Build history of the part. All positions in model axes, mm. A direction names the side the tool comes from. Round coordinates to 2 decimals unless told otherwise and drop trailing zeros. Order: outer loops, then holes, each group sorted by start corner. A loop starts at its lowest first (then second) coordinate and runs counter-clockwise, first axis right, second up. Notation, with made-up numbers: (-16, 48.25) -> (-1, 48.25) arc R22 cw to (-1, 84.25) -> close; hole circle Ø6 at (-5.5, -24.75). An arc over 180 degrees is marked (long way). Use a Markdown table: item, result. Add a question column.
Item 1: Slice it at B-B, the plane x = 64.4. Give the cut face in (y, z).
Item 2: Probe L1, parallel to X at y = 5.25, z = 0; L2, parallel to Z at x = 0, y = 7.15; L3, parallel to Z at x = -29, y = 5. List the from-to ranges inside material, lowest first.
Item 3: Slice it at C-C, the plane y = 2.5. State how many separate pieces and enclosed holes the cut face has, plus the area to 3 significant figures.
Item 4: Pin check, flat tips, straight feed: pin 1 (7 mm diameter, centred on x = 0, z = -64.4, fed in from -Y); pin 2 (1.5 mm diameter, centred on x = -7.5, y = 3.5, fed in from -Z); pin 3 (23 mm diameter, centred on x = 0, z = 0, fed in from +Y). Stop position of each tip, or through.
Item 5: Two-plate mould, pull along Z, no slides. Class faces 1 (the face through (-55.55, 4.19, 42.594)), 2 (the face through (32.06, 3.3, -31.58)): released by +Z, released by -Z, zero draft, split by the parting line, or undercut.
Item 6: 3-axis set-ups, long thin cutter, end or side, ignore diameter. For faces 3 (the face through (-0.566, 1.972, -60.087)), 4 (the face through (-46.23, 6.99, 35.44)), 5 (the face through (-38.6, 3.3, -39.18)): which of +Z, -Z, +X, -X, +Y, -Y reach the whole face in a straight line?
Item 7: Slice it at A-A, the plane z = 64.4. Give the cut face in (x, y), plus the area to 3 significant figures.
from build123d import *

# Parameters (mm, degrees)
SKETCH1_R           = 70
BOSS_EXTRUDE1_DEPTH = 6.5
SKETCH2_R           = 2.65
CUT_EXTRUDE1_DEPTH  = 7.5
SKETCH3_R           = 70
SKETCH3_R_2         = 58.25
SKETCH3_R_3         = 2.65
BOSS_EXTRUDE2_DEPTH = 2
CUT_EXTRUDE2_DEPTH  = 7.5
SKETCH5_R           = 2.65
CUT_EXTRUDE3_DEPTH  = 7.5
CUT_EXTRUDE4_DEPTH  = 4
SKETCH7_R           = 10
CUT_EXTRUDE5_DEPTH  = 7.5
CHAMFER1_SIZE       = 1
SKETCH8_R           = 4.35
CUT_EXTRUDE6_DEPTH  = 4


with BuildPart() as part:
    # Sketch1 → Boss-Extrude1 (new body)
    with BuildSketch(Plane(origin=(0, 0, 0), x_dir=(1, 0, 0), z_dir=(0, 1, 0))):
        Circle(SKETCH1_R)
    extrude(amount=BOSS_EXTRUDE1_DEPTH)

    # Sketch2 → Cut-Extrude1 (cut, through all)
    with BuildSketch(Plane(origin=(0, 6.5, 0), x_dir=(1, 0, 0), z_dir=(0, 1, 0))):
        with Locations((0, 64.4)):
            Circle(SKETCH2_R)
        with Locations((64.4, 0)):
            Circle(SKETCH2_R)
        with Locations((0, -64.4)):
            Circle(SKETCH2_R)
        with Locations((-64.4, 0)):
            Circle(SKETCH2_R)
    extrude(amount=-CUT_EXTRUDE1_DEPTH, mode=Mode.SUBTRACT)

    # Sketch3 → Boss-Extrude2 (add)
    with BuildSketch(Plane(origin=(0, 6.5, 0), x_dir=(1, 0, 0), z_dir=(0, 1, 0))):
        Circle(SKETCH3_R)
        Circle(SKETCH3_R_2, mode=Mode.SUBTRACT)
        with Locations((-64.4, 0)):
            Circle(SKETCH3_R_3, mode=Mode.SUBTRACT)
        with Locations((0, 64.4)):
            Circle(SKETCH3_R_3, mode=Mode.SUBTRACT)
        with Locations((64.4, 0)):
            Circle(SKETCH3_R_3, mode=Mode.SUBTRACT)
        with Locations((0, -64.4)):
            Circle(SKETCH3_R_3, mode=Mode.SUBTRACT)
    extrude(amount=BOSS_EXTRUDE2_DEPTH)

    # Sketch4 → Cut-Extrude2 (cut, through all)
    with BuildSketch(Plane(origin=(0, 6.5, 0), x_dir=(1, 0, 0), z_dir=(0, 1, 0))):
        with BuildLine():
            ThreePointArc((-13.305704258, 53.366264945), (-38.890872965, 38.890872965), (-53.366264945, 13.305704258))
            ThreePointArc((-53.366264945, 13.305704258), (-49.724395792, 7.244616149), (-43.663307682, 10.886485302))
            ThreePointArc((-43.663307682, 10.886485302), (-31.819805153, 31.819805153), (-10.886485302, 43.663307682))
            ThreePointArc((-10.886485302, 43.663307682), (-7.244616149, 49.724395792), (-13.305704258, 53.366264945))
        make_face()
        with BuildLine():
            ThreePointArc((43.663307682, 10.886485302), (31.819805153, 31.819805153), (10.886485302, 43.663307682))
            ThreePointArc((10.886485302, 43.663307682), (7.244616149, 49.724395792), (13.305704258, 53.366264945))
            ThreePointArc((13.305704258, 53.366264945), (38.890872965, 38.890872965), (53.366264945, 13.305704258))
            ThreePointArc((53.366264945, 13.305704258), (49.724395792, 7.244616149), (43.663307682, 10.886485302))
        make_face()
        with BuildLine():
            ThreePointArc((10.886485302, -43.663307682), (31.819805153, -31.819805153), (43.663307682, -10.886485302))
            ThreePointArc((43.663307682, -10.886485302), (49.724395792, -7.244616149), (53.366264945, -13.305704258))
            ThreePointArc((53.366264945, -13.305704258), (38.890872965, -38.890872965), (13.305704258, -53.366264945))
            ThreePointArc((13.305704258, -53.366264945), (7.244616149, -49.724395792), (10.886485302, -43.663307682))
        make_face()
        with BuildLine():
            ThreePointArc((-43.663307682, -10.886485302), (-31.819805153, -31.819805153), (-10.886485302, -43.663307682))
            ThreePointArc((-10.886485302, -43.663307682), (-7.244616149, -49.724395792), (-13.305704258, -53.366264945))
            ThreePointArc((-13.305704258, -53.366264945), (-38.890872965, -38.890872965), (-53.366264945, -13.305704258))
            ThreePointArc((-53.366264945, -13.305704258), (-49.724395792, -7.244616149), (-43.663307682, -10.886485302))
        make_face()
    extrude(amount=-CUT_EXTRUDE2_DEPTH, mode=Mode.SUBTRACT)

    # Sketch5 → Cut-Extrude3 (cut, through all)
    with BuildSketch(Plane(origin=(0, 6.5, 0), x_dir=(1, 0, 0), z_dir=(0, 1, 0))):
        with Locations((0, 36.02147888)):
            Circle(SKETCH5_R)
        with Locations((31.195515792, 18.01073944)):
            Circle(SKETCH5_R)
        with Locations((31.195515792, -18.01073944)):
            Circle(SKETCH5_R)
        with Locations((0, -36.02147888)):
            Circle(SKETCH5_R)
        with Locations((-31.195515792, -18.01073944)):
            Circle(SKETCH5_R)
        with Locations((-31.195515792, 18.01073944)):
            Circle(SKETCH5_R)
    extrude(amount=-CUT_EXTRUDE3_DEPTH, mode=Mode.SUBTRACT)

    # Sketch6 → Cut-Extrude4 (cut)
    with BuildSketch(Plane.XZ):
        Polygon((27.195515792, -20.320140517), (31.195515792, -22.629541594), (35.195515792, -20.320140517), (35.195515792, -15.701338363), (31.195515792, -13.391937286), (27.195515792, -15.701338363), align=None)
        Polygon((-4, -33.712077803), (-4, -38.330879957), (0, -40.640281034), (4, -38.330879957), (4, -33.712077803), (0, -31.402676726), align=None)
        Polygon((-31.195515792, -13.391937286), (-35.195515792, -15.701338363), (-35.195515792, -20.320140517), (-31.195515792, -22.629541594), (-27.195515792, -20.320140517), (-27.195515792, -15.701338363), align=None)
        Polygon((-27.195515792, 20.320140517), (-31.195515792, 22.629541594), (-35.195515792, 20.320140517), (-35.195515792, 15.701338363), (-31.195515792, 13.391937286), (-27.195515792, 15.701338363), align=None)
        Polygon((4, 33.712077803), (4, 38.330879957), (0, 40.640281034), (-4, 38.330879957), (-4, 33.712077803), (0, 31.402676726), align=None)
        Polygon((31.195515792, 13.391937286), (35.195515792, 15.701338363), (35.195515792, 20.320140517), (31.195515792, 22.629541594), (27.195515792, 20.320140517), (27.195515792, 15.701338363), align=None)
    extrude(amount=-CUT_EXTRUDE4_DEPTH, mode=Mode.SUBTRACT)

    # Sketch7 → Cut-Extrude5 (cut, through all)
    with BuildSketch(Plane(origin=(0, 6.5, 0), x_dir=(1, 0, 0), z_dir=(0, 1, 0))):
        Circle(SKETCH7_R)
    extrude(amount=-CUT_EXTRUDE5_DEPTH, mode=Mode.SUBTRACT)

    # Chamfer1
    chamfer1_edges = [part.edges().sort_by_distance(p)[0] for p in [
        (-58.25, 8.5, 0),
    ]]
    chamfer(chamfer1_edges, length=CHAMFER1_SIZE)

    # Sketch8 → Cut-Extrude6 (cut)
    with BuildSketch(Plane.XZ):
        with Locations((-64.4, 0)):
            Circle(SKETCH8_R)
        with Locations((0, 64.4)):
            Circle(SKETCH8_R)
        with Locations((64.4, 0)):
            Circle(SKETCH8_R)
        with Locations((0, -64.4)):
            Circle(SKETCH8_R)
    extrude(amount=-CUT_EXTRUDE6_DEPTH, mode=Mode.SUBTRACT)


solid = part.part
Check sheet entries:
| question | item | result |
|---|---|---|
| 1 | outline | (0, -27.43) -> (8.5, -27.43) -> (8.5, -2.65) -> (4, -2.65) -> (4, -4.35) -> (0, -4.35) -> close; (0, 4.35) -> (4, 4.35) -> (4, 2.65) -> (8.5, 2.65) -> (8.5, 27.43) -> (0, 27.43) -> close |
| 2 | L1 | -70 to -67.05, -61.75 to -10, 10 to 61.75, 67.05 to 70 |
| 2 | L2 | -70 to -67.05, -61.75 to -58.25, 58.25 to 61.75, 67.05 to 70 |
| 2 | L3 | -63.71 to -46.73, -34.41 to -19.49, -16.53 to 16.53, 19.49 to 34.41, 46.73 to 63.71 |
| 3 | separate pieces | 1 |
| 3 | enclosed holes | 15 |
| 3 | area | 12,000 mm2 |
| 4 | pin 1 | y = 4 |
| 4 | pin 2 | z = -69.67 |
| 4 | pin 3 | y = 6.5 |
| 5 | face 1 | split by the parting line |
| 5 | face 2 | undercut |
| 6 | face 3 | -Y |
| 6 | face 4 | +Y |
| 6 | face 5 | +Y, -Y |
| 7 | outline | (-27.43, 0) -> (-4.35, 0) -> (-4.35, 4) -> (-2.65, 4) -> (-2.65, 8.5) -> (-27.43, 8.5) -> close; (2.65, 4) -> (4.35, 4) -> (4.35, 0) -> (27.43, 0) -> (27.43, 8.5) -> (2.65, 8.5) -> close |
| 7 | area | 408 mm2 |
